Answer from the drawing. Dimensions are ordinates in mm from the lowest x, y and z of the part. Round coordinates to 2 decimals unless told otherwise and drop trailing zeros. Loops run counter-clockwise (first coordinate to the right, second up) from the corner with the lowest first, then second, coordinate; pieces in that order, holes last. Notation, with made-up numbers: (81, 40.25) - (97, 40.25) arc R13 cw to (97, 64.25) - close; hole circle Ø1 at (-12, -40). An arc over 180 degrees is marked (long way). Answer as CSV lines item,"result". Start each with the question number.
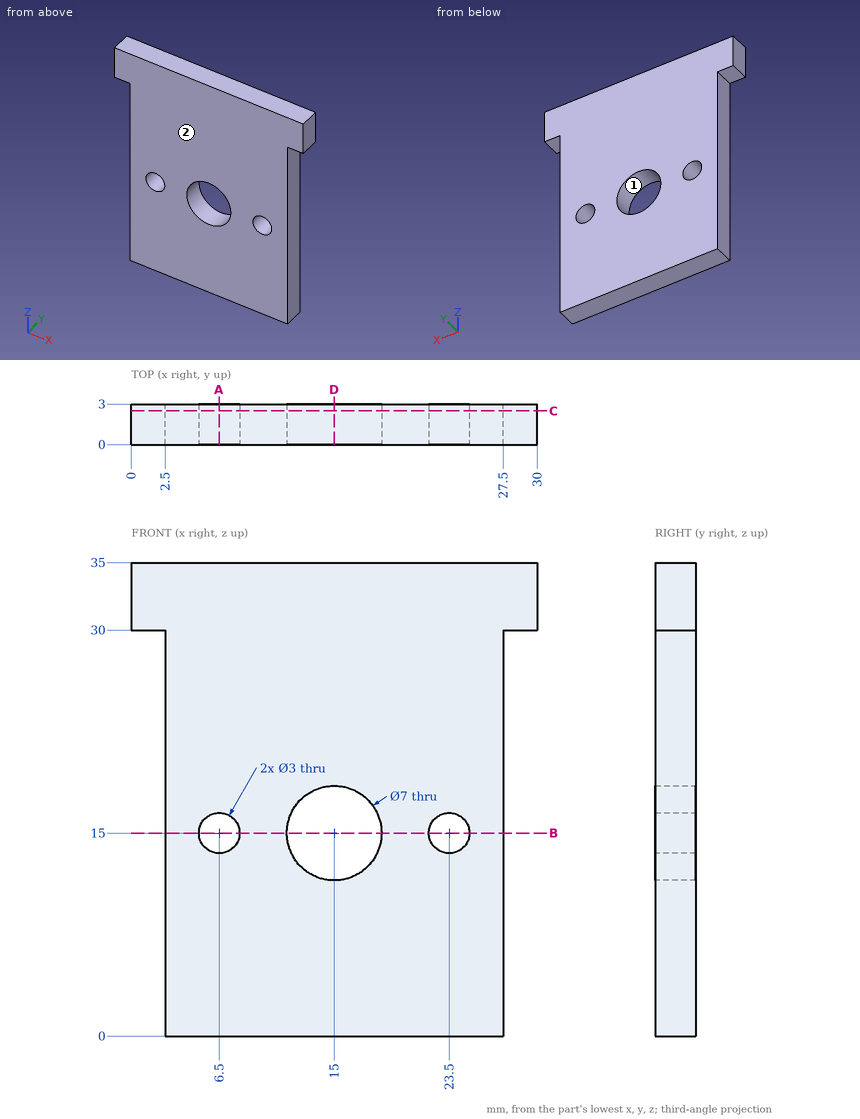
Item 1: Section A-A, the plane x = 6.5 is taken. Give the vertices of the cut face in (y, z), and give its area (3 significant figures).
Item 2: Flat-ended cylindrical pins translate along their axes: pin 1 Ø1.2 at (x, y) = (29, 2) entering from -Z; pin 2 Ø1.5 at (y, z) = (2.5, 14) entering from -X. Find the tip coordinate at first contact, or state that the pin passes through.
Item 3: Section C-C, the plane y = 2.5 is taken. Give the vertices of the cut face in (x, z).
Item 4: Find the intervals of material crossed by L1, parallel to X at y = 1.55, z = 15; L2, parallel to X at y = 1.45, z = 14; L3, parallel to X at y = 1.75, z = 9, in increasing order.
Item 5: Section D-D, the plane x = 15 is taken. Give the vertices of the cut face in (y, z).
Item 6: Determine the mould class of the marked faces 1 and 2 for opening direction X: pulls with the +X half, pulls with the -X half, needs draft (parallel to the pull), parting line crosses it, or undercut.
Item 7: Section B-B, the plane z = 15 is taken. Give the vertices of the cut face in (x, y), and give its area (3 significant figures).
Answer:
1,outline,"(0, 0) - (3, 0) - (3, 13.5) - (0, 13.5) - close; (0, 16.5) - (3, 16.5) - (3, 35) - (0, 35) - close"
1,area,"96.0 mm²"
2,pin 1,"stops at z = 30"
2,pin 2,"stops at x = 2.5"
3,outline,"(0, 30) - (2.5, 30) - (2.5, 0) - (27.5, 0) - (27.5, 30) - (30, 30) - (30, 35) - (0, 35) - close; hole circle Ø3 at (6.5, 15); hole circle Ø7 at (15, 15); hole circle Ø3 at (23.5, 15)"
4,L1,"x = 2.5 to 5, 8 to 11.5, 18.5 to 22, 25 to 27.5"
4,L2,"x = 2.5 to 5.38, 7.62 to 11.65, 18.35 to 22.38, 24.62 to 27.5"
4,L3,"x = 2.5 to 27.5"
5,outline,"(0, 0) - (3, 0) - (3, 11.5) - (0, 11.5) - close; (0, 18.5) - (3, 18.5) - (3, 35) - (0, 35) - close"
6,face 1,"undercut"
6,face 2,"needs draft"
7,outline,"(2.5, 0) - (5, 0) - (5, 3) - (2.5, 3) - close; (8, 0) - (11.5, 0) - (11.5, 3) - (8, 3) - close; (18.5, 0) - (22, 0) - (22, 3) - (18.5, 3) - close; (25, 0) - (27.5, 0) - (27.5, 3) - (25, 3) - close"
7,area,"36.0 mm²"
